Check sheet for the modelled part. Datum: model origin and axes. Units: mm. Coordinates: 2 decimals unless noted, no trailing zeros. Loops run counter-clockwise (first coordinate to the right, second up) from the corner with the lowest first, then second, coordinate; pieces in that order, holes last.
```python
from build123d import *

# Parameters (mm, degrees)
SKETCH_1_R               = 3.3
SKETCH_1_R_2             = 1.4
EXTRUDE_1_DEPTH          = 4
CUT_EXTRUDE_2_DEPTH      = 7.146543744
PATTERN_CIRCULAR_1_COUNT = 9


with BuildPart() as part:
    # 草图1 → 凸台-拉伸1 (new body)
    with BuildSketch(Plane.XY):
        Circle(SKETCH_1_R)
        Circle(SKETCH_1_R_2, mode=Mode.SUBTRACT)
    extrude(amount=EXTRUDE_1_DEPTH)

    # 草图1<3> → 切除-拉伸2 (cut, through all)
    with BuildSketch(Plane.XY):
        with BuildLine():
            Line((1.662533824, 0.311405332), (1.376068977, 0.25774827))
            ThreePointArc((1.376068977, 0.25774827), (1.394004406, 0.129428421), (1.4, 0))
            ThreePointArc((1.4, 0), (1.394004406, -0.129428421), (1.376068977, -0.25774827))
            Line((1.376068977, -0.25774827), (1.662533824, -0.311405332))
            add(Edge.make_bspline(
                [(1.662533824, -0.311405332), (1.675205333, -0.313778803), (1.711083832, -0.317659393), (1.780190094, -0.314430955), (1.890417179, -0.293797665), (2.027621966, -0.245157179), (2.149610149, -0.181207231), (2.236923472, -0.123298158), (2.286284468, -0.086512346), (2.298711222, -0.076985185)],
                knots=[0, 0, 0, 0, 0, 0.005604068, 0.015718248, 0.029959916, 0.048733667, 0.068727063, 0.075548145, 0.075548145, 0.075548145, 0.075548145, 0.075548145], degree=4))
            ThreePointArc((2.298711222, -0.076985185), (2.299677783, -0.038497986), (2.3, 0))
            ThreePointArc((2.3, 0), (2.299677783, 0.038497986), (2.298711222, 0.076985185))
            add(Edge.make_bspline(
                [(1.662533824, 0.311405332), (1.675205333, 0.313778803), (1.711083832, 0.317659393), (1.780190094, 0.314430955), (1.890417179, 0.293797665), (2.027621966, 0.245157179), (2.149610149, 0.181207231), (2.236923472, 0.123298158), (2.286284468, 0.086512346), (2.298711222, 0.076985185)],
                knots=[0, 0, 0, 0, 0, 0.005604068, 0.015718248, 0.029959916, 0.048733667, 0.068727063, 0.075548145, 0.075548145, 0.075548145, 0.075548145, 0.075548145], degree=4))
        make_face()
    cut_extrude_2 = extrude(amount=CUT_EXTRUDE_2_DEPTH, mode=Mode.SUBTRACT)

    # 阵列(圆周)1: 切除-拉伸2 ×9 about axis
    pattern_circular_1_axis = Axis((0, 0, 4), (0, 0, 1))
    for i in range(1, PATTERN_CIRCULAR_1_COUNT):
        add(cut_extrude_2.rotate(pattern_circular_1_axis, i * 360 / PATTERN_CIRCULAR_1_COUNT), mode=Mode.SUBTRACT)


solid = part.part
```
1) Section check B-B on x = -2. Give the number of separate pieces and of enclosed holes in the cut face, plus the area to 3 significant figures.
Answer sheet:
separate pieces: 3
enclosed holes: 0
area: 17.7 mm2
2) Section check C-C on x = 2.75. Enter the section's corners in (y, z), plus the area to 3 significant figures.
Answer sheet:
outline: (-1.82, 0) - (1.82, 0) - (1.82, 4) - (-1.82, 4) - close
area: 14.6 mm2
3) Scan lines: line 1 (X direction, y = -1.25, z = 1.15); line 2 (X direction, y = -1.75, z = 3.6); line 3 (Y direction, x = -0.25, z = 0.7). Record each from-to range of solid material in increasing order.
Answer sheet:
line 1: x = -3.05 to -1.07, 0.63 to 1.03, 1.76 to 3.05
line 2: x = -2.8 to -1.23, -0.66 to -0.01, 0.62 to 2.8
line 3: y = -3.29 to -1.38, 1.38 to 3.29
4) Section check A-A on y = 2.5. Enter the section's corners in (x, z).
Answer sheet:
outline: (-2.15, 0) - (2.15, 0) - (2.15, 4) - (-2.15, 4) - close
